Autodesk Inventor part; units mm, degrees
ref_plane "YZ Plane" through (0, 0, 0) normal (1, 0, 0) x (0, 1, 0)
ref_plane "XZ Plane" through (0, 0, 0) normal (0, 1, 0) x (-1, 0, 0)
ref_plane "XY Plane" through (0, 0, 0) normal (0, 0, 1) x (1, 0, 0)
sketch "スケッチ1" plane through (0, 0, 0) normal (0, 0, 1) x (1, 0, 0)
  line L0 (0, 0) -> (-15, 0)
  line L1 (-15, 0) -> (-15, -15)
  line L2 (-15, -15) -> (0, -15)
  line L3 (0, -15) -> (0, 0)
  line L4 (-13.5, -1.5) -> (-1.5, -1.5)
  line L5 (-1.5, -1.5) -> (-1.5, -13.5)
  line L6 (-1.5, -13.5) -> (-13.5, -13.5)
  line L7 (-13.5, -13.5) -> (-13.5, -1.5)
  dimension "d0" = 15
  dimension "d1" = 15
  dimension "d2" = 12
  dimension "d3" = 12
  dimension "d4" = 1.5
  dimension "d5" = 1.5
extrude "押し出し1" add sketch "スケッチ1" along normal blind 112
sketch "スケッチ2" plane through (0, -15, 0) normal (1, 0, 0) x (0, 0, -1)
  line L0 (0, 15) -> (-112, 15)
  line L1 (0, 0) -> (0, 15)
  line L2 (-112, 0) -> (-112, 15)
  point P0 (-106, 7.5)
  point P1 (-6, 7.5)
  dimension "d8" = 7.5
  dimension "d9" = 7.5
  dimension "d10" = 6
  dimension "d11" = 6
hole "穴1" at (0, -7.5, 106) at (0, -7.5, 6) direction (-1, 0, 0) diameter 3 end through all
sketch "スケッチ3" plane through (-15, -15, 0) normal (0, -1, 0) x (1, 0, 0)
  line L0 (0, 0) -> (0, 112)
  line L1 (0, 112) -> (15, 112)
  line L2 (0, 0) -> (15, 0)
  point P0 (7.5, 97)
  point P1 (7.5, 15)
  dimension "d19" = 7.5
  dimension "d20" = 7.5
  dimension "d21" = 15
  dimension "d22" = 15
hole "穴2" at (-7.5, -15, 97) at (-7.5, -15, 15) direction (0, 1, 0) diameter 3 end through all
sketch "スケッチ4" plane through (-15, 0, 0) normal (0, 1, 0) x (1, 0, 0)
  line L0 (15, 0) -> (0, 0)
  line L1 (0, 0) -> (0, -112)
  line L2 (15, -112) -> (0, -112)
  circle A0 centre (7.5, -97) radius 1.5
  circle A1 centre (7.5, -15) radius 1.5
  point P0 (7.5, -7.5)
  point P1 (7.5, -104.5)
  point P2 (7.5, -76.5)
  point P3 (7.5, -56)
  point P4 (7.5, -35.5)
  dimension "d30" = 7.5
  dimension "d31" = 7.5
  dimension "d32" = 7.5
  dimension "d33" = 7.5
  dimension "d34" = 7.5
  dimension "d35" = 7.5
  dimension "d36" = 82
  dimension "d37" = 7.5
  dimension "d38" = 20.5
  dimension "d39" = 20.5
  dimension "d40" = 20.5
hole "穴3" at (-7.5, 0, 7.5) at (-7.5, 0, 104.5) at (-7.5, 0, 76.5) at (-7.5, 0, 56) at (-7.5, 0, 35.5) direction (0, -1, 0) diameter 7.5 end through all
sketch "スケッチ5" plane through (0, -15, 0) normal (1, 0, 0) x (0, 0, -1)
  circle A0 centre (-106, 7.5) radius 1.5
  circle A1 centre (-6, 7.5) radius 1.5
  line L0 (-106, 7.5) -> (-6, 7.5)
  point P0 (0, 15)
  point P1 (-97, 7.5)
  point P2 (-88, 7.5)
  point P3 (-79, 7.5)
  point P4 (-70, 7.5)
  point P5 (-61, 7.5)
  dimension "d48" = 100
  dimension "d51" = 9
  dimension "d56" = 9
hole "穴4" at (0, -7.5, 97) at (0, -7.5, 88) at (0, -7.5, 79) at (0, -7.5, 70) at (0, -7.5, 61) direction (-1, 0, 0) diameter 7.5 end through all
equation "\"d1\" = d0"
equation "\"d3\" = d2"
equation "\"d5\" = d4"
properties part number "前後直動12x12_3" material "アルミニウム 6061"
Input: part model. Units: mm. Frame: model coordinates. A direction names the side the tool comes from. Give positions to 0.01 mm unless a question says otherwise; leave off trailing zeros. Order: outer loops, then holes, each group sorted by start corner. A loop starts at its lowest first (then second) coordinate and runs counter-clockwise, first axis right, second up. Notation, with made-up numbers: (25.25, 11) - (64.25, 11) arc R16 cw to (64.25, 36) - close; hole circle Ø9 at (45.5, -21). An arc over 180 degrees is marked (long way). Put each result on its own line as item: value.
Item 1: Section query B-B, the plane z = 40.5. Return loops of the section in (x, y).
Found:
outline: (-15, -15) - (0, -15) - (0, 0) - (-15, 0) - close; hole (-13.5, -13.5) - (-1.5, -13.5) - (-1.5, -1.5) - (-13.5, -1.5) - close
Item 2: Section query C-C, the plane z = 76.5. Return loops of the section in (x, y).
Found:
outline: (-15, -15) - (-11.25, -15) - (-11.25, -13.5) - (-13.5, -13.5) - (-13.5, -10.3) - (-15, -10.3) - close; (-15, -4.7) - (-13.5, -4.7) - (-13.5, -1.5) - (-11.25, -1.5) - (-11.25, 0) - (-15, 0) - close; (-3.75, -15) - (0, -15) - (0, -10.3) - (-1.5, -10.3) - (-1.5, -13.5) - (-3.75, -13.5) - close; (-3.75, -1.5) - (-1.5, -1.5) - (-1.5, -4.7) - (0, -4.7) - (0, 0) - (-3.75, 0) - close
Item 3: Section query A-A, the plane z = 88. Return loops of the section in (x, y), then the cut area to 3 significant figures.
Found:
outline: (-15, -15) - (0, -15) - (0, -11.25) - (-1.5, -11.25) - (-1.5, -13.5) - (-13.5, -13.5) - (-13.5, -11.25) - (-15, -11.25) - close; (-15, -3.75) - (-13.5, -3.75) - (-13.5, -1.5) - (-1.5, -1.5) - (-1.5, -3.75) - (0, -3.75) - (0, 0) - (-15, 0) - close
area: 58.5 mm^2
Item 4: Contact query for a flat-ended pin moving along its axis: pin 1 (6 mm diameter, centred on y = -7.5, z = 79, fed in from +X). Output: stop coordinate, or through.
Found:
pin 1: passes through
Item 5: Access query for faces 1 (the flat face through (-1.5, -7, 55)), 2 (the cylindrical face through (-0.76, -8.626, 84.423)). Directions: +Z, -Z, +X, -X, +Y, -Y. A direction counts if a zero-diameter tool reaches every point of the face in a straight line with its end or side. Return the directions, or none.
Found:
face 1: +Z, -Z
face 2: +X, -X
Item 6: Ray query, L1, parallel to Y at x = -4, z = 47; L2, parallel to Y at x = -14.1, z = 70. Return the intervals inside material, ascending. Write a range as from..to.
Found:
L1: y = -15..-13.5, -1.5..0
L2: y = -15..-11.25, -3.75..0
Item 7: Section query D-D, the plane x = -7.5. Count the separate pieces of the cut face and the enclosed holes in it, then the cut area to 4 significant figures.
Found:
separate pieces: 16
enclosed holes: 0
area: 205.5 mm^2
Item 8: Draft query along Z for faces 3 (the flat face through (-12, -1.5, 55)), 4 (the cylindrical face through (-0.76, -8.626, 75.423)), 5 (the flat face through (-1, -7, 112)). Return one class per face: +Z half, -Z half, draft (parallel to the pull), parting line (faces both ways), or undercut.
Found:
face 3: draft
face 4: undercut
face 5: +Z half
